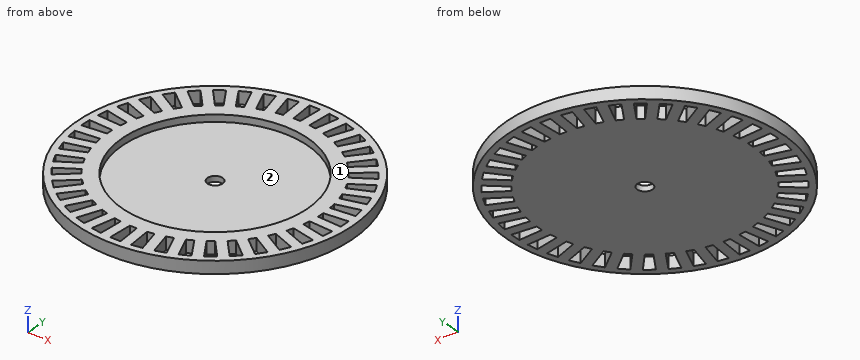
```python
from build123d import *

# Parameters (mm, degrees)
F0_R     = 20
F0_R_2   = 13.45
F1_DEPTH = 1.8
F0_R_3   = 1.1
F2_DEPTH = 0.8


with BuildPart() as f1:
    # F0 (on Top) → F1 (new body)
    with BuildSketch(Plane.XY):
        Circle(F0_R)
        Polygon((-10.553413, -15.827023), (-11.791209, -14.927711), (-9.571323, -12.221773), (-8.762306, -12.809558), align=None, mode=Mode.SUBTRACT)
        Polygon((-14.927711, -11.791209), (-15.827023, -10.553413), (-12.879604, -8.665895), (-12.291819, -9.474912), align=None, mode=Mode.SUBTRACT)
        Polygon((-12.899375, -13.981248), (-13.981248, -12.899375), (-11.365391, -10.574017), (-10.658284, -11.281124), align=None, mode=Mode.SUBTRACT)
        Polygon((-7.947591, -17.283083), (-9.310831, -16.588478), (-7.541578, -13.568587), (-6.650571, -14.022578), align=None, mode=Mode.SUBTRACT)
        Polygon((-5.146073, -18.313577), (-6.60119, -17.840781), (-5.326134, -14.581298), (-4.375077, -14.890315), align=None, mode=Mode.SUBTRACT)
        Polygon((-2.217842, -18.89313), (-3.729005, -18.653785), (-2.979543, -15.234969), (-1.991854, -15.391403), align=None, mode=Mode.SUBTRACT)
        Polygon((-16.588478, -9.310831), (-17.283083, -7.947591), (-14.07668, -6.544389), (-13.622689, -7.435396), align=None, mode=Mode.SUBTRACT)
        Polygon((-17.840781, -6.60119), (-18.313577, -5.146073), (-14.927141, -4.261739), (-14.618124, -5.212796), align=None, mode=Mode.SUBTRACT)
        Polygon((-18.653785, -3.729005), (-18.89313, -2.217842), (-15.410046, -1.874151), (-15.253611, -2.861839), align=None, mode=Mode.SUBTRACT)
        Polygon((0.765, -19.007471), (-0.765, -19.007471), (-0.559585, -15.513504), (0.440415, -15.513504), align=None, mode=Mode.SUBTRACT)
        Polygon((3.729005, -18.653785), (2.217842, -18.89313), (1.874151, -15.410046), (2.861839, -15.253611), align=None, mode=Mode.SUBTRACT)
        Polygon((6.60119, -17.840781), (5.146073, -18.313577), (4.261739, -14.927141), (5.212796, -14.618124), align=None, mode=Mode.SUBTRACT)
        Polygon((9.310831, -16.588478), (7.947591, -17.283083), (6.544389, -14.07668), (7.435396, -13.622689), align=None, mode=Mode.SUBTRACT)
        Polygon((11.791209, -14.927711), (10.553413, -15.827023), (8.665895, -12.879604), (9.474912, -12.291819), align=None, mode=Mode.SUBTRACT)
        Polygon((13.981248, -12.899375), (12.899375, -13.981248), (10.574017, -11.365391), (11.281124, -10.658284), align=None, mode=Mode.SUBTRACT)
        Polygon((15.827023, -10.553413), (14.927711, -11.791209), (12.221773, -9.571323), (12.809558, -8.762306), align=None, mode=Mode.SUBTRACT)
        Polygon((17.283083, -7.947591), (16.588478, -9.310831), (13.568587, -7.541578), (14.022578, -6.650571), align=None, mode=Mode.SUBTRACT)
        Polygon((18.313577, -5.146073), (17.840781, -6.60119), (14.581298, -5.326134), (14.890315, -4.375077), align=None, mode=Mode.SUBTRACT)
        Polygon((18.89313, -2.217842), (18.653785, -3.729005), (15.234969, -2.979543), (15.391403, -1.991854), align=None, mode=Mode.SUBTRACT)
        Polygon((-19.007471, -0.765), (-19.007471, 0.765), (-15.513504, 0.559585), (-15.513504, -0.440415), align=None, mode=Mode.SUBTRACT)
        Polygon((-18.89313, 2.217842), (-18.653785, 3.729005), (-15.234969, 2.979543), (-15.391403, 1.991854), align=None, mode=Mode.SUBTRACT)
        Polygon((-18.313577, 5.146073), (-17.840781, 6.60119), (-14.581298, 5.326134), (-14.890315, 4.375077), align=None, mode=Mode.SUBTRACT)
        Polygon((-17.283083, 7.947591), (-16.588478, 9.310831), (-13.568587, 7.541578), (-14.022578, 6.650571), align=None, mode=Mode.SUBTRACT)
        Polygon((-15.827023, 10.553413), (-14.927711, 11.791209), (-12.221773, 9.571323), (-12.809558, 8.762306), align=None, mode=Mode.SUBTRACT)
        Polygon((-13.981248, 12.899375), (-12.899375, 13.981248), (-10.574017, 11.365391), (-11.281124, 10.658284), align=None, mode=Mode.SUBTRACT)
        Polygon((-11.791209, 14.927711), (-10.553413, 15.827023), (-8.665895, 12.879604), (-9.474912, 12.291819), align=None, mode=Mode.SUBTRACT)
        Polygon((-9.310831, 16.588478), (-7.947591, 17.283083), (-6.544389, 14.07668), (-7.435396, 13.622689), align=None, mode=Mode.SUBTRACT)
        Polygon((-6.60119, 17.840781), (-5.146073, 18.313577), (-4.261739, 14.927141), (-5.212796, 14.618124), align=None, mode=Mode.SUBTRACT)
        Polygon((-3.729005, 18.653785), (-2.217842, 18.89313), (-1.874151, 15.410046), (-2.861839, 15.253611), align=None, mode=Mode.SUBTRACT)
        Circle(F0_R_2, mode=Mode.SUBTRACT)
        Polygon((19.007471, 0.765), (19.007471, -0.765), (15.513504, -0.559585), (15.513504, 0.440415), align=None, mode=Mode.SUBTRACT)
        Polygon((18.653785, 3.729005), (18.89313, 2.217842), (15.410046, 1.874151), (15.253611, 2.861839), align=None, mode=Mode.SUBTRACT)
        Polygon((17.840781, 6.60119), (18.313577, 5.146073), (14.927141, 4.261739), (14.618124, 5.212796), align=None, mode=Mode.SUBTRACT)
        Polygon((16.588478, 9.310831), (17.283083, 7.947591), (14.07668, 6.544389), (13.622689, 7.435396), align=None, mode=Mode.SUBTRACT)
        Polygon((-0.765, 19.007471), (0.765, 19.007471), (0.559585, 15.513504), (-0.440415, 15.513504), align=None, mode=Mode.SUBTRACT)
        Polygon((2.217842, 18.89313), (3.729005, 18.653785), (2.979543, 15.234969), (1.991854, 15.391403), align=None, mode=Mode.SUBTRACT)
        Polygon((5.146073, 18.313577), (6.60119, 17.840781), (5.326134, 14.581298), (4.375077, 14.890315), align=None, mode=Mode.SUBTRACT)
        Polygon((7.947591, 17.283083), (9.310831, 16.588478), (7.541578, 13.568587), (6.650571, 14.022578), align=None, mode=Mode.SUBTRACT)
        Polygon((12.899375, 13.981248), (13.981248, 12.899375), (11.365391, 10.574017), (10.658284, 11.281124), align=None, mode=Mode.SUBTRACT)
        Polygon((14.927711, 11.791209), (15.827023, 10.553413), (12.879604, 8.665895), (12.291819, 9.474912), align=None, mode=Mode.SUBTRACT)
        Polygon((10.553413, 15.827023), (11.791209, 14.927711), (9.571323, 12.221773), (8.762306, 12.809558), align=None, mode=Mode.SUBTRACT)
    extrude(amount=F1_DEPTH)

    # F0 (on Top) → F2 (join)
    with BuildSketch(Plane.XY):
        Circle(F0_R_2)
        Circle(F0_R_3, mode=Mode.SUBTRACT)
    extrude(amount=F2_DEPTH)


solid = f1.part
```
Input: part model. Units: mm. Frame: model coordinates. Face numbers are marked on the shaded views. Coordinates: 2 decimals unless noted, no trailing zeros. Use a Markdown table: item, result.
1) Contact query for flat-ended pins moving along their axis: pin 1 (0.5 mm diameter, centred on x = 0, z = 0.5, fed in from +Y); pin 2 (3 mm diameter, centred on x = 0, y = 0, fed in from +Z); pin 3 (0.5 mm diameter, centred on x = 0.5, z = 1, fed in from -Y). Output: stop coordinate, or through.
Results found:
| item | result |
|---|---|
| pin 1 | stops at y = 20 |
| pin 2 | stops at z = 0.8 |
| pin 3 | stops at y = -20 |
2) Material intervals for line 1 along Y through (x, z) = (0, 1.45); line 2 along Y through (x, z) = (0, 0.4); line 3 along X through (y, z) = (10.5, 0.95), sorted ascending. Write a range as from..to.
Results found:
| item | result |
|---|---|
| line 1 | y = -20..-19.01, -15.51..-13.45, 13.45..15.51, 19.01..20 |
| line 2 | y = -20..-19.01, -15.51..-1.1, 1.1..15.51, 19.01..20 |
| line 3 | x = -17.02..-15.74, -13.35..-8.41, 8.41..13.46, 15.74..17.02 |
3) Cut plane A-A (z = 1.5). Give the number of separate pieces and of enclosed holes in the cut face, then the cut area to 3 significant figures.
Results found:
| item | result |
|---|---|
| separate pieces | 1 |
| enclosed holes | 41 |
| area | 512 mm2 |
4) Pull-direction query (X, two-part tool) for the marked faces 1 and 2; classes: released by +X, released by -X, zero draft, split by the parting line, or undercut.
Results found:
| item | result |
|---|---|
| face 1 | zero draft |
| face 2 | undercut |
